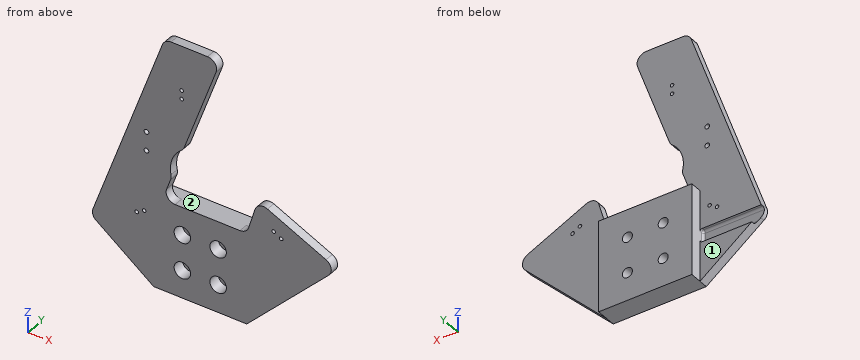
from build123d import *

# Parameters (mm, degrees)
SKETCH1_W                       = 65
SKETCH1_H                       = 64
EXTRUDE1_DEPTH                  = 8.255
EXTRUDE2_DEPTH                  = 6.35
FILLET1_R                       = 6.35
CBORE_FOR_M6_SBHCS1_D           = 7
CBORE_FOR_M6_SBHCS1_CBORE_D     = 11.5
CBORE_FOR_M6_SBHCS1_CBORE_DEPTH = 8.38
M3X0_5_TAPPED_HOLE1_D           = 2.5
M4X0_7_TAPPED_HOLE1_D           = 3.3
SKETCH10_W                      = 45.157529952
SKETCH10_H                      = 9.398
CUT_EXTRUDE1_DEPTH              = 3.175
FILLET2_R                       = 1.5875
SKETCH11_R                      = 20.588537239
CUT_EXTRUDE2_DEPTH              = 173.088346863
FILLET3_R                       = 6.35


with BuildPart() as part:
    # Sketch1 → Extrude1 (new body)
    with BuildSketch(Plane(origin=(0, 0, 0), x_dir=(1, 0, 0), z_dir=(0, 1, 0))):
        Rectangle(SKETCH1_W, SKETCH1_H)
    extrude(amount=EXTRUDE1_DEPTH)

    # Sketch3 → Extrude2 (add)
    with BuildSketch(Plane.XZ):
        Polygon((-32.5, -32), (-76.484147351, 1.251326619), (-24.877631504, 145.512128668), (14.112838434, 145.512128668), (-26.493933355, 32), (32.5, 32), (40.26552936, 58.115798324), (96.00808235, 32), (32.5, -32), align=None)
    extrude(amount=EXTRUDE2_DEPTH)

    # Fillet1
    fillet1_edges = [part.edges().sort_by_distance(p)[0] for p in [
        (96.00808235, -3.175, 32),
        (40.26552936, -3.175, 58.115798324),
        (32.5, -3.175, 32),
        (-26.493933355, -3.175, 32),
        (-76.484147351, -3.175, 1.251326619),
        (-24.877631504, -3.175, 145.512128668),
        (14.112838434, -3.175, 145.512128668),
    ]]
    fillet(fillet1_edges, radius=FILLET1_R)

    # CBORE for M6 SBHCS1 (through all)
    with Locations(Plane.XZ.offset(6.35)):
        with Locations((-12.5, 12.5), (12.5, 12.5), (12.5, -12.5), (-12.5, -12.5)):
            CounterBoreHole(CBORE_FOR_M6_SBHCS1_D / 2, CBORE_FOR_M6_SBHCS1_CBORE_D / 2, CBORE_FOR_M6_SBHCS1_CBORE_DEPTH)

    # M3x0.5 Tapped Hole1 (through all)
    with Locations(Plane.XZ.offset(6.35)):
        with Locations((-12.991981474, 114.259500014), (-12.991981474, 108.259500014), (51.311236439, 40.865980186), (56.507388862, 37.865980186), (-39.204872739, 18.874519842), (-44.401025162, 15.874519842)):
            Hole(M3X0_5_TAPPED_HOLE1_D / 2)

    # M4x0.7 Tapped Hole1 (through all)
    with Locations(Plane(origin=(0, 0, 0), x_dir=(-1, 0, 0), z_dir=(0, 1, 0))):
        with Locations((37.535205925, 75.138578877), (37.535205925, 61.868858743)):
            Hole(M4X0_7_TAPPED_HOLE1_D / 2)

    # Sketch10 → Cut-Extrude1 (cut)
    with BuildSketch(Plane(origin=(0, 0, 0), x_dir=(1, 0, 0), z_dir=(0, 1, 0))):
        with Locations((-55.078764976, -0.003190653)):
            Rectangle(SKETCH10_W, SKETCH10_H)
    extrude(amount=-CUT_EXTRUDE1_DEPTH, mode=Mode.SUBTRACT)

    # Fillet2
    fillet2_edges = [part.edges().sort_by_distance(p)[0] for p in [
        (-50.558701218, -3.175, -4.695809347),
        (-32.5, -3.175, 0.003190653),
        (-32.5, -1.5875, -4.695809347),
        (-53.835070304, -3.175, 4.702190653),
        (-32.5, -1.5875, 4.702190653),
    ]]
    fillet(fillet2_edges, radius=FILLET2_R)

    # Sketch11 → Cut-Extrude2 (cut, through all)
    with BuildSketch(Plane(origin=(0, 0, 0), x_dir=(-1, 0, 0), z_dir=(0, 1, 0))):
        with Locations((0.295205925, 56.000000014)):
            Circle(SKETCH11_R)
    extrude(amount=-CUT_EXTRUDE2_DEPTH, mode=Mode.SUBTRACT)

    # Fillet3
    fillet3_edges = [part.edges().sort_by_distance(p)[0] for p in [
        (-20.019691254, -3.175, 50.098089803),
        (-11.80057866, -3.175, 73.07378881),
    ]]
    fillet(fillet3_edges, radius=FILLET3_R)


solid = part.part
The model under review builds one solid part; all positions refer to its coordinate system, in mm. Face numbers are marked on the shaded views. Coordinates: 2 decimals unless noted, no trailing zeros. Write each loop counter-clockwise with the first axis right and the second up, starting at its lowest first coordinate (ties: lowest second). Pieces come first, ordered by that corner, then holes. Notation, with made-up numbers: (16, -32) -> (31, -32) arc R7 cw to (31, -23) -> close; hole circle Ø8 at (87, -27.5). An arc over 180 degrees is marked (long way). Answer in a Markdown table with one row per item.
1. Draft analysis for pull direction X (two halves, no side actions). For the marked faces 1 and 2, state which applies: +X half, -X half, draft (parallel to the pull), parting line (faces both ways), or undercut.
Answers below:
| item | result |
|---|---|
| face 1 | draft |
| face 2 | undercut |
2. We need section C-C, the plane z = -12.5. State the section outline as (x, y) points (3 decimals).
Answers below:
| item | result |
|---|---|
| outline | (-58.294, -6.35) -> (-18.25, -6.35) -> (-18.25, 2.03) -> (-16, 2.03) -> (-16, 8.255) -> (-32.5, 8.255) -> (-32.5, 0) -> (-58.294, 0) -> close; (-9, 2.03) -> (-6.75, 2.03) -> (-6.75, -6.35) -> (6.75, -6.35) -> (6.75, 2.03) -> (9, 2.03) -> (9, 8.255) -> (-9, 8.255) -> close; (16, 2.03) -> (18.25, 2.03) -> (18.25, -6.35) -> (51.85, -6.35) -> (51.85, 0) -> (32.5, 0) -> (32.5, 8.255) -> (16, 8.255) -> close |
3. Wall thickness on probe 1 along Z at (x, y) = (12, -1.5); probe 2 along Z at (x, y) = (23.5, 3); probe 3 along Y at (x, z) = (-47.5, 54.5): over which ranges is each line inside the solid? List them lowest first. Write a range as [from, to].
Answers below:
| item | result |
|---|---|
| probe 1 | z = [-32, -18.23], [-6.77, 6.77], [18.23, 32] |
| probe 2 | z = [-32, 32] |
| probe 3 | y = [-6.35, 0] |
4. We need section B-B, the plane x = 22.5. State the section outline as (y, z) points (3 decimals).
Answers below:
| item | result |
|---|---|
| outline | (-6.35, -32) -> (8.255, -32) -> (8.255, 32) -> (-6.35, 32) -> close |
5. We need section D-D, the plane z = 85. State the section outline as (x, y) points.
Answers below:
| item | result |
|---|---|
| outline | (-46.52, -6.35) -> (-7.53, -6.35) -> (-7.53, 0) -> (-46.52, 0) -> close |
6. Clearance check with flat-ended pins moving along their axes: pin 1 Ø8 at (x, z) = (-44.5, -11.5) entering from +Y; pin 2 Ø2 at (x, z) = (-12.99, 114.26) entering from -Y; pin 3 Ø1 at (x, y) = (14.5, -4.5) entering from +Z; pin 4 Ø8 at (x, z) = (12.5, 12.5) entering from -Y. State where each tip first meets the part, or that it passes through.
Answers below:
| item | result |
|---|---|
| pin 1 | stops at y = 0 |
| pin 2 | passes through |
| pin 3 | stops at z = 32 |
| pin 4 | stops at y = 2.03 |
7. We need section A-A, the plane z = 12.5. State the section outline as (x, y) points (3 decimals).
Answers below:
| item | result |
|---|---|
| outline | (-72.46, -6.35) -> (-18.25, -6.35) -> (-18.25, 2.03) -> (-16, 2.03) -> (-16, 8.255) -> (-32.5, 8.255) -> (-32.5, 0) -> (-72.46, 0) -> close; (-9, 2.03) -> (-6.75, 2.03) -> (-6.75, -6.35) -> (6.75, -6.35) -> (6.75, 2.03) -> (9, 2.03) -> (9, 8.255) -> (-9, 8.255) -> close; (16, 2.03) -> (18.25, 2.03) -> (18.25, -6.35) -> (76.658, -6.35) -> (76.658, 0) -> (32.5, 0) -> (32.5, 8.255) -> (16, 8.255) -> close |
